Geometry: see drawing. Coordinates: mm, zero at the bounding-box minimum. A direction names the side the tool comes from. Round coordinates to 2 decimals unless told otherwise and drop trailing zeros. Write each loop counter-clockwise with the first axis right and the second up, starting at its lowest first coordinate (ties: lowest second). Pieces come first, ordered by that corner, then holes. Notation, with made-up numbers: (-38.75, 7.5) -> (-4.75, 7.5) arc R28 cw to (-4.75, 40.5) -> close; hole circle Ø5 at (2, 5). An arc over 180 degrees is marked (long way). Use CSV: the item, a comma, the result in double quotes.
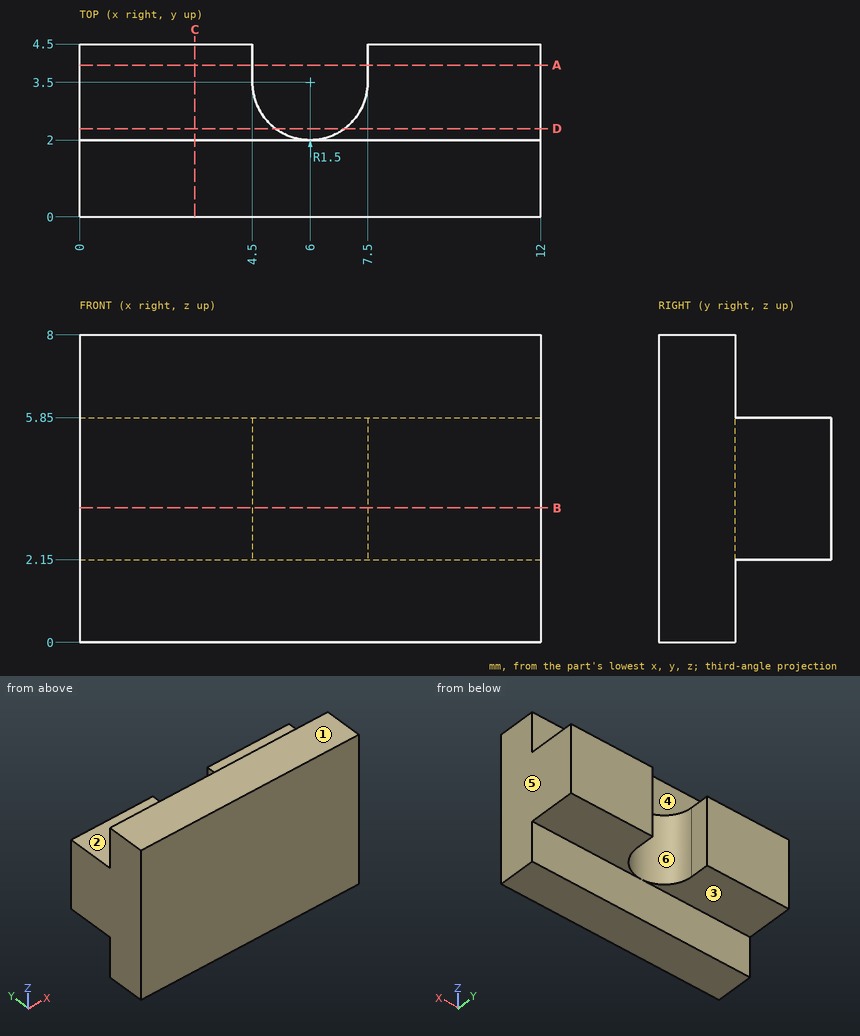
Item 1: Pull-direction query (X, two-part tool) for the marked faces 4, 5 and 6; classes: +X half, -X half, draft (parallel to the pull), parting line (faces both ways), or undercut.
Worked answers:
face 4,"draft"
face 5,"+X half"
face 6,"undercut"
Item 2: Set-up query: the marked faces 1, 2 and 3. Return all of +Z, -Z, +X, -X, +Y, -Y with unobstructed straight access to the full face (end or side cutting, diameter ignored); none if empty.
Worked answers:
face 1,"+Z, +X, -X, +Y, -Y"
face 2,"+Z, +X, -X, +Y"
face 3,"-Z, +X, -X, +Y"
Item 3: Section query C-C on x = 3. Return the cut outline in (y, z), plus the area to 4 significant figures.
Worked answers:
outline,"(0, 0) -> (2, 0) -> (2, 2.15) -> (4.5, 2.15) -> (4.5, 5.85) -> (2, 5.85) -> (2, 8) -> (0, 8) -> close"
area,"25.25 mm²"
Item 4: Section query A-A on y = 3.95. Return the cut outline in (x, z).
Worked answers:
outline,"(0, 2.15) -> (4.5, 2.15) -> (4.5, 5.85) -> (0, 5.85) -> close; (7.5, 2.15) -> (12, 2.15) -> (12, 5.85) -> (7.5, 5.85) -> close"
Item 5: First-contact query: pin 1 Ø0.6 at (x, z) = (7, 1.5) entering from +Y; pin 2 Ø1.2 at (x, y) = (3.5, 3.5) entering from +Z. Flat tips, straight axial feed; report the tip coordinate or a pass-through.
Worked answers:
pin 1,"stops at y = 2"
pin 2,"stops at z = 5.85"
Item 6: Section query D-D on y = 2.3. Return the cut outline in (x, z), plus the area to 3 significant figures.
Worked answers:
outline,"(0, 2.15) -> (5.1, 2.15) -> (5.1, 5.85) -> (0, 5.85) -> close; (6.9, 2.15) -> (12, 2.15) -> (12, 5.85) -> (6.9, 5.85) -> close"
area,"37.7 mm²"
Item 7: Section query B-B on z = 3.5. Return the cut outline in (x, y).
Worked answers:
outline,"(0, 0) -> (12, 0) -> (12, 4.5) -> (7.5, 4.5) -> (7.5, 3.5) arc R1.5 cw to (4.5, 3.5) -> (4.5, 4.5) -> (0, 4.5) -> close"
Item 8: Line query: line 1 (Y direction, x = 6.25, z = 7.75); line 2 (Z direction, x = 11.25, y = 2.45); line 3 (X direction, y = 3.4, z = 5). Output: solid intervals per line, ascending.
Worked answers:
line 1,"y = 0 to 2"
line 2,"z = 2.15 to 5.85"
line 3,"x = 0 to 4.5, 7.5 to 12"
